```python
from build123d import *

# Parameters (mm, degrees)
CYLINDER056_R     = 1.6
CYLINDER056_DEPTH = 10
CYLINDER057_R     = 5
CYLINDER057_DEPTH = 25
BOX014_W          = 79
BOX014_H          = 10
BOX014_DEPTH      = 29
BOX015_W          = 3
BOX015_H          = 3
BOX015_DEPTH      = 44
BOX016_W          = 3
BOX016_H          = 3
BOX016_DEPTH      = 44
BOX017_W          = 101
BOX017_H          = 15
BOX017_DEPTH      = 3
BOX013_W          = 99
BOX013_H          = 60
BOX013_DEPTH      = 128
EXTRUDE017_DEPTH  = 111


with BuildPart() as cono001:
    # Cone001 → Cone001 (revolve)
    with BuildSketch(Plane(origin=(0, 0, -96), x_dir=(1, 0, 0), z_dir=(0, -1, 0))):
        Polygon((0, 0), (1.6, 0), (4.1, 3), (0, 3), align=None)
    revolve(axis=Axis((0, 0, -96), (0, 0, 1)))


with BuildPart() as cilindro056:
    # Cylinder056 → Cylinder056 (new body)
    with BuildSketch(Plane.XY.offset(-106)):
        Circle(CYLINDER056_R)
    extrude(amount=CYLINDER056_DEPTH)


with BuildPart() as fusion037:
    # Fusion037 base: copy of Cilindro056
    add(cilindro056.part)

    # Fusion037: union Cono001
    add(cono001.part)


with BuildPart() as fusion037_1:
    # Fusion037 placement: moved
    add(fusion037.part.moved(Location((202, -62, 0))))


with BuildPart() as fusion038:
    # Fusion038 base: copy of Cilindro056
    add(cilindro056.part)

    # Fusion038: union Cono001
    add(cono001.part)


with BuildPart() as fusion038_1:
    # Fusion038 placement: moved
    add(fusion038.part.moved(Location((240, -83, 0))))


with BuildPart() as fusion039:
    # Fusion039 base: copy of Cilindro056
    add(cilindro056.part)

    # Fusion039: union Cono001
    add(cono001.part)


with BuildPart() as fusion039_1:
    # Fusion039 placement: moved
    add(fusion039.part.moved(Location((280, -62, 0))))


with BuildPart() as cilindro057:
    # Cylinder057 → Cylinder057 (new body)
    with BuildSketch(Plane(origin=(266, -119, -70), x_dir=(1, 0, 0), z_dir=(0, 1, 0))):
        Circle(CYLINDER057_R)
    extrude(amount=CYLINDER057_DEPTH)


with BuildPart() as fusion040:
    # Box014 → Box014 (new body)
    with BuildSketch(Plane(origin=(202, -112, -39), x_dir=(1, 0, 0), z_dir=(0, 0, 1))):
        with Locations((39.5, 5)):
            Rectangle(BOX014_W, BOX014_H)
    extrude(amount=BOX014_DEPTH)

    # Fusion040: union Fusion037, Fusion038, Fusion039, Cilindro057
    add(fusion037_1.part)
    add(fusion038_1.part)
    add(fusion039_1.part)
    add(cilindro057.part)


with BuildPart() as cubo014:
    # Box015 → Box015 (new body)
    with BuildSketch(Plane(origin=(289, -96, -55), x_dir=(1, 0, 0), z_dir=(0, 0, 1))):
        with Locations((1.5, 1.5)):
            Rectangle(BOX015_W, BOX015_H)
    extrude(amount=BOX015_DEPTH)


with BuildPart() as cubo015:
    # Box016 → Box016 (new body)
    with BuildSketch(Plane(origin=(191, -96, -55), x_dir=(1, 0, 0), z_dir=(0, 0, 1))):
        with Locations((1.5, 1.5)):
            Rectangle(BOX016_W, BOX016_H)
    extrude(amount=BOX016_DEPTH)


with BuildPart() as cubo016:
    # Box017 → Box017 (new body)
    with BuildSketch(Plane(origin=(191, -108, -58), x_dir=(1, 0, 0), z_dir=(0, 0, 1))):
        with Locations((50.5, 7.5)):
            Rectangle(BOX017_W, BOX017_H)
    extrude(amount=BOX017_DEPTH)


with BuildPart() as cubo012:
    # Box013 → Box013 (new body)
    with BuildSketch(Plane(origin=(132, 23, -93), x_dir=(1, 0, 0), z_dir=(0, 0, 1))):
        with Locations((49.5, 30)):
            Rectangle(BOX013_W, BOX013_H)
    extrude(amount=BOX013_DEPTH)


with BuildPart() as soporte_lcd:
    # Sketch013 → Extrude017 (new body)
    with BuildSketch(Plane.YZ.offset(126)):
        Polygon((18, 26), (18, -99), (78, -99), (78, -79), (38, 26), align=None)
    extrude(amount=EXTRUDE017_DEPTH)

    # Cut016: cut Cubo012
    add(cubo012.part, mode=Mode.SUBTRACT)


with BuildPart() as soporte_lcd_1:
    # Cut016 placement: moved
    add(soporte_lcd.part.moved(Location((60, -130, 0))))

    # Fusion041: union Cubo014, Cubo015, Cubo016
    add(cubo014.part)
    add(cubo015.part)
    add(cubo016.part)

    # Cut017: cut Fusion040
    add(fusion040.part, mode=Mode.SUBTRACT)


solid = soporte_lcd_1.part
```
Part model, mm, in its own coordinate system. A direction names the side the tool comes from. Round coordinates to 2 decimals unless told otherwise and drop trailing zeros. Order: outer loops, then holes, each group sorted by start corner. A loop starts at its lowest first (then second) coordinate and runs counter-clockwise, first axis right, second up. Notation, with made-up numbers: M 6,81 L 17,81 A23 cw 17,119 Z; hole C -11.75,79.25 d5. An arc over 180 degrees is marked long. Put each result on its own line as item: value. Start each with the question number.
1. Drop flat-ended pins along their axis: pin 1 (2 mm diameter, centred on x = 218.5, z = -51, fed in from +Y); pin 2 (1.6 mm diameter, centred on x = 193, y = -94.5, fed in from +Z); pin 3 (11 mm diameter, centred on x = 259.5, y = -102, fed in from +Z); pin 4 (6 mm diameter, centred on x = 265.5, y = -58.5, fed in from +Z). Give the stop position or say it passes through.
2. Drill centre lines: probe 1 along Z at (x, y) = (288.5, -103); probe 2 along Y at (x, z) = (202, -97); probe 3 along X at (y, z) = (-88.5, -70.5). Where is each one in solid material? Low to high. Write a range as [from, to].
3. Slice it at C-C on x = 266. List the corners of the cut face in (y, z), then the cut area to 3 significant figures.
4. Slice it at A-A on x = 233. List the corners of the cut face in (y, z), then the cut area to 3 significant figures.
5. Slice it at B-B on y = -62. List the corners of the cut face in (x, z), then the cut area to 3 significant figures.
6. Two-plate mould, pull along Y, no slides. Class faces 1 (the face through (203.526, -61.519, -97.521)), 2 (the face through (293.96, -71.72, -27.23)), 3 (the face through (241, -112, -50)): +Y half, -Y half, draft (parallel to the pull), parting line (faces both ways), or undercut.
7. Slice it at D-D on z = -73.5. List the corners of the cut face in (x, y), then the cut area to 3 significant figures.
8. Tool access for faces 4 (the face through (194, -95, -33)), 5 (the face through (241, -73, -93)), 6 (the face through (241, -109, -10)): list every direction of +Z, -Z, +X, -X, +Y, -Y with a clear straight run to the whole face (end or side of a thin tool).
Findings:
1. pin 1: y = -107
1. pin 2: z = -11
1. pin 3: z = 26
1. pin 4: z = -93
2. probe 1: [-99, -93], [-58, -55]
2. probe 2: [-112, -63.6], [-60.4, -52]
2. probe 3: [186, 192], [291, 297]
3. outline: M -112,-99 L -52,-99 L -52,-93 L -107,-93 L -107,-75 L -112,-75 Z; M -112,-65 L -107,-65 L -107,-58 L -93,-58 L -93,-55 L -107,-55 L -107,-39 L -112,-39 Z; M -112,-10 L -107,-10 L -107,26 L -112,26 Z
3. area: 802 mm2
4. outline: M -112,-99 L -52,-99 L -52,-93 L -107,-93 L -107,-58 L -93,-58 L -93,-55 L -107,-55 L -107,-39 L -112,-39 Z; M -112,-10 L -107,-10 L -107,26 L -112,26 Z
4. area: 852 mm2
5. outline: M 186,-99 L 200.4,-99 L 200.4,-96 L 197.9,-93 L 192,-93 L 192,-52.75 L 186,-52.75 Z; M 203.6,-99 L 278.4,-99 L 278.4,-96 L 275.9,-93 L 206.1,-93 L 203.6,-96 Z; M 281.6,-99 L 297,-99 L 297,-52.75 L 291,-52.75 L 291,-93 L 284.1,-93 L 281.6,-96 Z
5. area: 1,100 mm2
6. face 1: undercut
6. face 2: +Y half
6. face 3: -Y half
7. outline: M 186,-112 L 262.43,-112 L 262.43,-107 L 192,-107 L 192,-54.1 L 186,-54.1 Z; M 269.57,-112 L 297,-112 L 297,-54.1 L 291,-54.1 L 291,-107 L 269.57,-107 Z
7. area: 1,150 mm2
8. face 4: +Z, +Y
8. face 5: +Y
8. face 6: +Y, -Y
